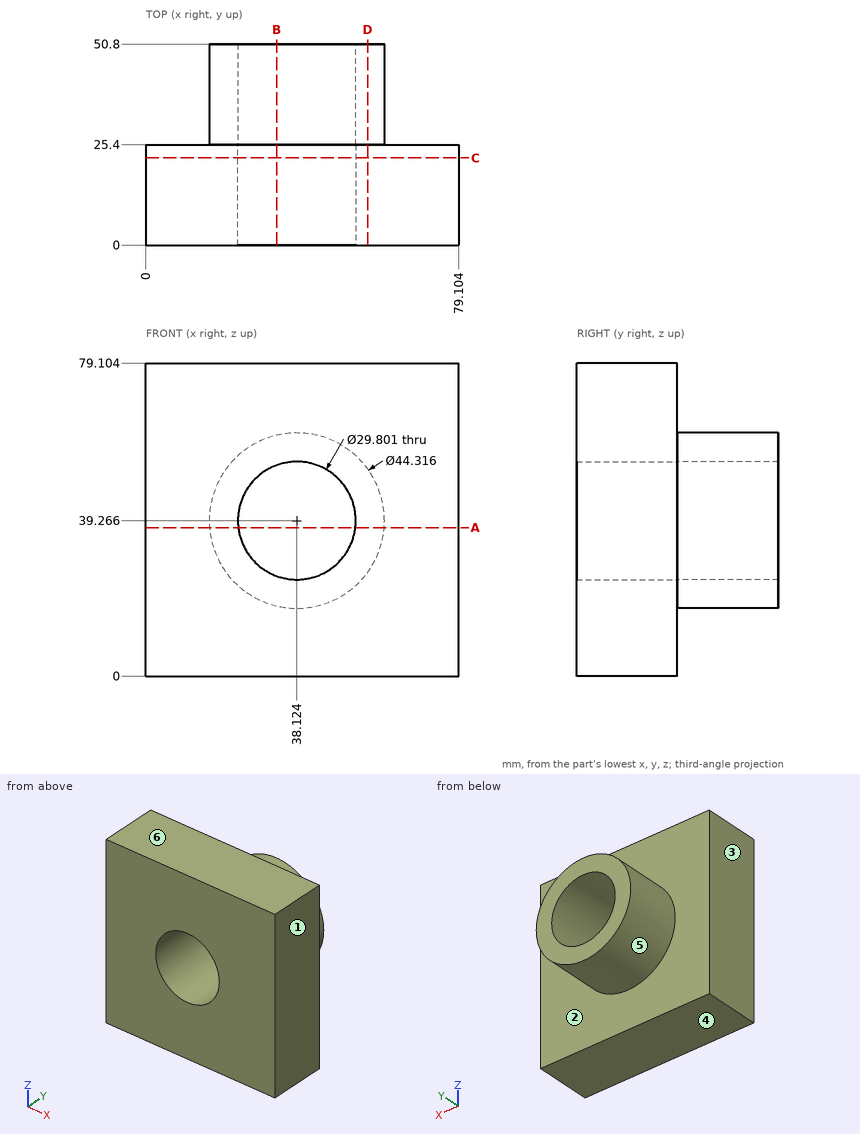
Design review of the part shown in the three views and the two pictorial views. Dimensions are in mm from the part's minimum x, y and z. A direction names the side the tool comes from. Round coordinates to 2 decimals unless told otherwise and drop trailing zeros. Loops run counter-clockwise (first coordinate to the right, second up) from the corner with the lowest first, then second, coordinate; pieces in that order, holes last. Notation, with made-up numbers: (-8.5, 9.5) - (36.5, 9.5) arc R13 ccw to (36.5, 19.5) - close; hole circle Ø3 at (61.5, 23.5). An arc over 180 degrees is marked (long way). Use CSV: the item, a comma, the result in double quotes.
(1) For line 1 (Y direction, x = 24, z = 58.5); line 2 (Z direction, x = 36, y = 44) (1 decimal); line 3 (X direction, y = 18.5, z = 48.5) (1 decimal), list the stretches that pass through material, from the lowest coordinate up.
Working result:
line 1,"y = 0 to 25.4"
line 2,"z = 17.2 to 24.5, 54 to 61.3"
line 3,"x = 0 to 26.4, 49.8 to 79.1"
(2) Clearance check with flat-ended pins moving along their axes: P1, Ø1, axis at x = 27.5, y = 36.5, coming from the +Z side; P2, Ø1.5, axis at y = 28.5, z = 25.5, coming from the -X side; P3, Ø12, axis at x = 34, y = 45.5, coming from the +Z side. State where each tip first meets the part, or that it passes through.
Working result:
P1,"stops at z = 58.98"
P2,"stops at x = 20.19"
P3,"stops at z = 61.42"
(3) Machinability: for the marked faces 1 and 2, which of the approach directions +Z, -Z, +X, -X, +Y, -Y give a long, thin tool a straight path to every point of the face, cutting with its end or side? Answer none if there is none.
Working result:
face 1,"+Z, -Z, +X, +Y, -Y"
face 2,"+Y"
(4) Take a section at C-C, the plane y = 22. Give the boundary of the cut face in (x, z) (1 decimal).
Working result:
outline,"(0, 0) - (79.1, 0) - (79.1, 79.1) - (0, 79.1) - close; hole circle Ø29.8 at (38.1, 39.3)"
(5) Take a section at A-A, the plane z = 37.5. Give the boundary of the cut face in (x, y).
Working result:
outline,"(0, 0) - (23.33, 0) - (23.33, 50.8) - (16.04, 50.8) - (16.04, 25.4) - (0, 25.4) - close; (52.92, 0) - (79.1, 0) - (79.1, 25.4) - (60.21, 25.4) - (60.21, 50.8) - (52.92, 50.8) - close"
(6) Take a section at D-D, the plane x = 56. Give the boundary of the cut face in (y, z).
Working result:
outline,"(0, 0) - (25.4, 0) - (25.4, 26.17) - (50.8, 26.17) - (50.8, 52.36) - (25.4, 52.36) - (25.4, 79.1) - (0, 79.1) - close"
(7) The part is to be moulded in two halves that separate along Z. For the marked faces 3, 4, 5 and 6, say which applies: pulls with the +Z half, pulls with the -Z half, needs draft (parallel to the pull), parting line crosses it, or undercut.
Working result:
face 3,"needs draft"
face 4,"pulls with the -Z half"
face 5,"parting line crosses it"
face 6,"pulls with the +Z half"
(8) Take a section at B-B, the plane x = 33. Give the boundary of the cut face in (y, z) (1 decimal), plus the area to 3 significant figures.
Working result:
outline,"(0, 0) - (25.4, 0) - (25.4, 17.7) - (50.8, 17.7) - (50.8, 25.3) - (0, 25.3) - close; (0, 53.3) - (50.8, 53.3) - (50.8, 60.8) - (25.4, 60.8) - (25.4, 79.1) - (0, 79.1) - close"
area,"1,680 mm^2"
